```python
from build123d import *

# Parameters (mm, degrees)
F1_DEPTH = 25.4
F3_DEPTH = 25.4


# Not quite as in the source:
# - the program builds the solid bodies; features that only make, move or delete a surface that nothing else refers to are left out


with BuildPart() as f1:
    # F0 (on Front) → F1 (new body)
    with BuildSketch(Plane.XZ):
        with BuildLine():
            Line((9.6126659133, 12.4514792114), (-12.6748333757, 12.4514792114))
            ThreePointArc((-12.6748333757, 12.4514792114), (-20.2182408326, 4.9080717545), (-27.7616482896, 12.4514792114))
            Line((-27.7616482896, 12.4514792114), (-27.861725539, 12.4514792114))
            Line((-27.861725539, 12.4514792114), (-27.861725539, -11.4652235061))
            Line((-27.861725539, -11.4652235061), (27.8617236763, -11.4652235061))
            Line((27.8617236763, -11.4652235061), (27.8617236763, 12.2047088224))
            ThreePointArc((27.8617236763, 12.2047088224), (18.6154667795, 3.3261161383), (9.6126659133, 12.4514792114))
        make_face()
        with BuildLine():
            Line((-12.6748333757, 12.4514792114), (-17.7898686341, 12.4514792114))
            ThreePointArc((-17.7898686341, 12.4514792114), (-20.2182408326, 10.0231070129), (-22.6466130312, 12.4514792114))
            Line((-22.6466130312, 12.4514792114), (-27.7616482896, 12.4514792114))
            ThreePointArc((-27.7616482896, 12.4514792114), (-20.2182408326, 4.9080717545), (-12.6748333757, 12.4514792114))
        make_face()
    extrude(amount=F1_DEPTH)

    # F0 (on Front) → F3 (join)
    with BuildSketch(Plane.XZ):
        with BuildLine():
            ThreePointArc((-22.6466130312, 12.4514792114), (-20.2182408326, 14.87985141), (-17.7898686341, 12.4514792114))
            Line((-17.7898686341, 12.4514792114), (-12.6748333757, 12.4514792114))
            ThreePointArc((-12.6748333757, 12.4514792114), (-16.8959093658, 19.2238576479), (-24.8351495055, 18.4169758688))
            ThreePointArc((-24.8351495055, 18.4169758688), (-24.460861538, 17.8481513463), (-24.3295943797, 17.1800033439))
            ThreePointArc((-24.3295943797, 17.1800033439), (-25.2407357632, 15.634657994), (-27.0340151871, 15.6838492415))
            ThreePointArc((-27.0340151871, 15.6838492415), (-27.5774921245, 14.1081072584), (-27.7616482896, 12.4514792114))
            Line((-27.7616482896, 12.4514792114), (-22.6466130312, 12.4514792114))
        make_face()
        with BuildLine():
            Line((-12.6748333757, 12.4514792114), (-17.7898686341, 12.4514792114))
            ThreePointArc((-17.7898686341, 12.4514792114), (-20.2182408326, 10.0231070129), (-22.6466130312, 12.4514792114))
            Line((-22.6466130312, 12.4514792114), (-27.7616482896, 12.4514792114))
            ThreePointArc((-27.7616482896, 12.4514792114), (-20.2182408326, 4.9080717545), (-12.6748333757, 12.4514792114))
        make_face()
        with BuildLine():
            Line((9.6126659133, 12.4514792114), (-12.6748333757, 12.4514792114))
            ThreePointArc((-12.6748333757, 12.4514792114), (-20.2182408326, 4.9080717545), (-27.7616482896, 12.4514792114))
            Line((-27.7616482896, 12.4514792114), (-27.861725539, 12.4514792114))
            Line((-27.861725539, 12.4514792114), (-27.861725539, -11.4652235061))
            Line((-27.861725539, -11.4652235061), (27.8617236763, -11.4652235061))
            Line((27.8617236763, -11.4652235061), (27.8617236763, 12.2047088224))
            ThreePointArc((27.8617236763, 12.2047088224), (18.6154667795, 3.3261161383), (9.6126659133, 12.4514792114))
        make_face()
        with BuildLine():
            ThreePointArc((27.8650605952, 12.4514792114), (18.7388632542, 21.5776765524), (9.6126659133, 12.4514792114))
            Line((9.6126659133, 12.4514792114), (27.8617236763, 12.4514792114))
            Line((27.8617236763, 12.4514792114), (27.8617236763, 12.2047088224))
            ThreePointArc((27.8617236763, 12.2047088224), (27.8642263273, 12.3280827367), (27.8650605952, 12.4514792114))
        make_face()
        with BuildLine():
            Line((27.8617236763, 12.4514792114), (9.6126659133, 12.4514792114))
            ThreePointArc((9.6126659133, 12.4514792114), (18.6154667795, 3.3261161383), (27.8617236763, 12.2047088224))
            Line((27.8617236763, 12.2047088224), (27.8617236763, 12.4514792114))
        make_face()
        with BuildLine():
            ThreePointArc((-24.3295943797, 17.1800033439), (-24.460861538, 17.8481513463), (-24.8351495055, 18.4169758688))
            ThreePointArc((-24.8351495055, 18.4169758688), (-26.0956599593, 17.1800033439), (-27.0340151871, 15.6838492415))
            ThreePointArc((-27.0340151871, 15.6838492415), (-25.2407357632, 15.634657994), (-24.3295943797, 17.1800033439))
        make_face()
        with BuildLine():
            ThreePointArc((-27.0340151871, 15.6838492415), (-26.0956599593, 17.1800033439), (-24.8351495055, 18.4169758688))
            ThreePointArc((-24.8351495055, 18.4169758688), (-27.4716836828, 18.2870473105), (-27.0340151871, 15.6838492415))
        make_face()
    extrude(amount=F3_DEPTH)


solid = f1.part
```
Source: CAD feature listing. Evaluate the final solid. Frame: model axes, mm. A direction names the side the tool comes from. Give positions to 0.01 mm unless a question says otherwise; leave off trailing zeros. Loops run counter-clockwise (first coordinate to the right, second up) from the corner with the lowest first, then second, coordinate; pieces in that order, holes last. Notation, with made-up numbers: (-34.75, -14.75) -> (7.25, -14.75) arc R16 cw to (7.25, 10.25) -> close; hole circle Ø8 at (55.25, 49.25). An arc over 180 degrees is marked (long way). Use a Markdown table: item, result. Add a question column.
(1) Access query for faces 1 (the face through (-1, -13, 12.451)), 2 (the face through (-27.862, -13, 1)). Directions: +Z, -Z, +X, -X, +Y, -Y. A direction counts if a zero-diameter tool reaches every point of the face in a straight line with its end or side. Return the directions, or none.
(2) Section query B-B (y = -2.25). Output: boundary loops of the cut face in (x, z).
(3) Ray query, line 1 (X direction, y = -1, z = 12.5); line 2 (X direction, y = -19, z = 13.5); line 3 (X direction, y = -24, z = -6). Return the intervals inside material, ascending.
(4) Section query C-C (z = 17). Output: boundary loops of the cut face in (x, y), then the cut area to 3 significant figures.
(5) Section query A-A (z = 11). Output: boundary loops of the cut face in (x, y).
(6) First-contact query: pin 1 Ø4 at (y, z) = (-5.5, -3) entering from +X; pin 2 Ø3 at (x, z) = (16.5, 16) entering from +Y; pin 3 Ø6.5 at (x, y) = (-5, -18.5) entering from +Z; pin 4 Ø1 at (x, y) = (15.5, -5) entering from +Z. Flat tips, straight axial feed; report the tip coordinate or a pass-through.
(7) Pull-direction query (Z, two-part tool) for faces 3 (the face through (0, -25.4, 2)), 4 (the face through (-27.572, -12.522, 14.131)), 5 (the face through (-16.79, -12.52, 19.17)); classes: +Z half, -Z half, draft (parallel to the pull), parting line (faces both ways), or undercut.
(8) Section query D-D (x = -1). Output: boundary loops of the cut face in (y, z), then the cut area to 3 significant figures.
Checked values:
| question | item | result |
|---|---|---|
| 1 | face 1 | +Z, +Y, -Y |
| 1 | face 2 | +Z, -Z, -X, +Y, -Y |
| 2 | outline | (-27.86, -11.47) -> (27.86, -11.47) -> (27.86, 12.2) arc R9.13 ccw (long way) to (9.61, 12.45) -> (-12.67, 12.45) arc R7.54 ccw to (-24.84, 18.42) arc R1.77 ccw (long way) to (-27.03, 15.68) arc R7.54 ccw to (-27.76, 12.45) -> (-27.86, 12.45) -> close; hole circle Ø4.86 at (-20.22, 12.45) |
| 3 | line 1 | -27.76 to -22.65, -17.79 to -12.67, 9.61 to 27.86 |
| 3 | line 2 | -27.69 to -22.41, -18.03 to -12.75, 9.67 to 27.8 |
| 3 | line 3 | -27.86 to 27.86 |
| 4 | outline | (-27.85, -25.4) -> (-14.2, -25.4) -> (-14.2, 0) -> (-27.85, 0) -> close; (10.83, -25.4) -> (26.65, -25.4) -> (26.65, 0) -> (10.83, 0) -> close |
| 4 | area | 749 mm^2 |
| 5 | outline | (-27.86, -25.4) -> (-22.17, -25.4) -> (-22.17, 0) -> (-27.86, 0) -> close; (-18.27, -25.4) -> (27.86, -25.4) -> (27.86, 0) -> (-18.27, 0) -> close |
| 6 | pin 1 | x = 27.86 |
| 6 | pin 2 | y = 0 |
| 6 | pin 3 | z = 12.45 |
| 6 | pin 4 | z = 21.16 |
| 7 | face 3 | draft |
| 7 | face 4 | undercut |
| 7 | face 5 | +Z half |
| 8 | outline | (-25.4, -11.47) -> (0, -11.47) -> (0, 12.45) -> (-25.4, 12.45) -> close |
| 8 | area | 607 mm^2 |
